```python
from build123d import *

# Parameters (mm, degrees)
SKETCH_1_R          = 1.25
EXTRUDE_1_DEPTH     = 2.5
SKETCH_2_R          = 2.25
CUT_EXTRUDE_1_DEPTH = 1
SCALE_1_SCALE       = 0.6


with BuildPart() as part:
    # 草图1 → 凸台-拉伸1 (new body)
    with BuildSketch(Plane.XY):
        with BuildLine():
            Line((-13, 3), (13, 3))
            ThreePointArc((13, 3), (16, 0), (13, -3))
            Line((13, -3), (-13, -3))
            ThreePointArc((-13, -3), (-16, 0), (-13, 3))
        make_face()
        with Locations((5, 0)):
            Circle(SKETCH_1_R, mode=Mode.SUBTRACT)
        with Locations((-5, 0)):
            Circle(SKETCH_1_R, mode=Mode.SUBTRACT)
    extrude(amount=EXTRUDE_1_DEPTH)

    # 草图2 → 切除-拉伸1 (cut)
    with BuildSketch(Plane.XY.offset(2.5)):
        with Locations((-5, 0)):
            Circle(SKETCH_2_R)
        with Locations((5, 0)):
            Circle(SKETCH_2_R)
    extrude(amount=-CUT_EXTRUDE_1_DEPTH, mode=Mode.SUBTRACT)


with BuildPart() as part_1:
    # 缩放比例1: scaled about (0, 0, 0)
    add(part.part.scale(SCALE_1_SCALE))


solid = part_1.part
```
Input: part model. Units: mm. Frame: model coordinates. A direction names the side the tool comes from. Round coordinates to 2 decimals unless told otherwise and drop trailing zeros. Order: outer loops, then holes, each group sorted by start corner. A loop starts at its lowest first (then second) coordinate and runs counter-clockwise, first axis right, second up. Notation, with made-up numbers: (-14.75, 27) - (40.25, 27) arc R22 ccw to (40.25, 35) - close; hole circle Ø4 at (9.25, 45). An arc over 180 degrees is marked (long way). One line per question, with ' | ' between items. Start each with the question number.
1) Cut plane C-C, the plane y = -1. Return the cut outline in (x, z).
2) Contact query for a flat-ended pin moving along its axis: P1, Ø1.6, axis at x = 3, y = 0, coming from the +Z side. Output: stop coordinate, or through.
3) Set-up query: faces 1 (the cylindrical face through (4.247, -0.517, 1.204)), 2 (the flat face through (0, 0, 0)). Return all of +Z, -Z, +X, -X, +Y, -Y with unobstructed straight access to the full face (end or side cutting, diameter ignored); none if empty.
4) Cut plane D-D, the plane x = -2.5. Return the cut outline in (y, z).
5) Cut plane B-B, the plane y = 0. Return the cut outline in (x, z), then the cut area to 3 significant figures.
6) Ray query, probe 1 along Y at (x, z) = (3, 0.3); probe 2 along Y at (x, z) = (3, 1.3); probe 3 along X at (y, z) = (0.25, 0.1). Return the intervals inside material, ascending.
7) Pull-direction query (X, two-part tool) for faces 3 (the cylindrical face through (-1.712, 0.406, 1.204)), 4 (the cylindrical face through (-9.6, 0, 0.7)), 5 (the cylindrical face through (9.6, 0, 0.7)); classes: +X half, -X half, draft (parallel to the pull), parting line (faces both ways), or undercut.
8) Cut plane A-A, the plane x = 3. Return the cut outline in (y, z), then the cut area to 3 significant figures.
Worked out:
1) outline: (-9.3, 0) - (9.3, 0) - (9.3, 1.5) - (3.91, 1.5) - (3.91, 0.9) - (2.09, 0.9) - (2.09, 1.5) - (-2.09, 1.5) - (-2.09, 0.9) - (-3.91, 0.9) - (-3.91, 1.5) - (-9.3, 1.5) - close
2) P1: stops at z = 0.9
3) face 1: +Z | face 2: -Z, +X, -X, +Y, -Y
4) outline: (-1.8, 0) - (-0.56, 0) - (-0.56, 0.9) - (-1.25, 0.9) - (-1.25, 1.5) - (-1.8, 1.5) - close; (0.56, 0) - (1.8, 0) - (1.8, 1.5) - (1.25, 1.5) - (1.25, 0.9) - (0.56, 0.9) - close
5) outline: (-9.6, 0) - (-3.75, 0) - (-3.75, 0.9) - (-4.35, 0.9) - (-4.35, 1.5) - (-9.6, 1.5) - close; (-2.25, 0) - (2.25, 0) - (2.25, 0.9) - (1.65, 0.9) - (1.65, 1.5) - (-1.65, 1.5) - (-1.65, 0.9) - (-2.25, 0.9) - close; (3.75, 0) - (9.6, 0) - (9.6, 1.5) - (4.35, 1.5) - (4.35, 0.9) - (3.75, 0.9) - close | area: 22.9 mm^2
6) probe 1: y = -1.8 to -0.75, 0.75 to 1.8 | probe 2: y = -1.8 to -1.35, 1.35 to 1.8 | probe 3: x = -9.58 to -3.71, -2.29 to 2.29, 3.71 to 9.58
7) face 3: undercut | face 4: -X half | face 5: +X half
8) outline: (-1.8, 0) - (-0.75, 0) - (-0.75, 0.9) - (-1.35, 0.9) - (-1.35, 1.5) - (-1.8, 1.5) - close; (0.75, 0) - (1.8, 0) - (1.8, 1.5) - (1.35, 1.5) - (1.35, 0.9) - (0.75, 0.9) - close | area: 2.43 mm^2
